Verification items for this drawing (mm, ordinates from the low corner). A direction names the side the tool comes from. Round coordinates to 2 decimals unless told otherwise and drop trailing zeros. Write each loop counter-clockwise with the first axis right and the second up, starting at its lowest first coordinate (ties: lowest second). Pieces come first, ordered by that corner, then holes.
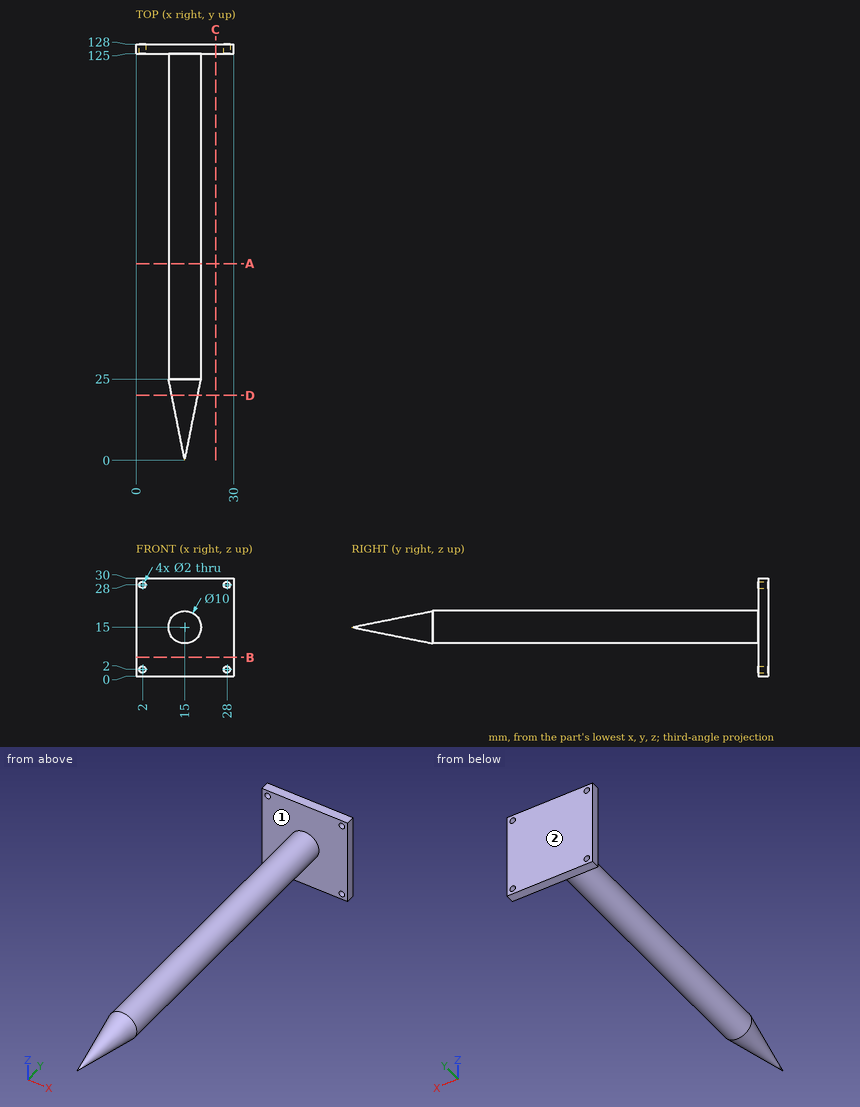
1. Section check B-B (z = 5.75). Record the cut outline in (x, y).
2. Section check C-C (x = 24.5). Record the cut outline in (y, z).
3. Scan lines: line 1 along Z through (x, y) = (28, 125.7); line 2 along Z through (x, y) = (15.25, 36). Record each from-to range of solid material in increasing order.
4. Section check D-D (y = 20). Record the cut outline in (x, z).
5. Section check A-A (y = 60.5). Record the cut outline in (x, z), plus the area to 3 significant figures.
6. Depth check by flat-ended pin: pin 1 Ø5 at (x, z) = (8.5, 22) entering from -Y; pin 2 Ø1.8 at (x, z) = (2, 2) entering from -Y; pin 3 Ø10 at (x, y) = (16, 21.5) entering from +Z; pin 4 Ø1.5 at (y, z) = (38, 15.5) entering from -X. Enter the tip coordinate at first touch or a pass-through.
7. Access from +Z, -Z, +X, -X, +Y, -Y to the whole of each face (thin tool, end or side, straight path). Record for the marked faces 1 and 2.
Results below:
1. outline: (0, 125) - (30, 125) - (30, 128) - (0, 128) - close
2. outline: (125, 0) - (128, 0) - (128, 30) - (125, 30) - close
3. line 1: z = 0 to 1, 3 to 27, 29 to 30
3. line 2: z = 10.01 to 19.99
4. outline: circle Ø8 at (15, 15)
5. outline: circle Ø10 at (15, 15)
5. area: 78.5 mm2
6. pin 1: stops at y = 125
6. pin 2: passes through
6. pin 3: stops at z = 20
6. pin 4: stops at x = 10
7. face 1: -Y
7. face 2: +Z, -Z, +X, -X, +Y
